Input: part model. Units: mm. Frame: model coordinates. Face numbers are marked on the shaded views. A direction names the side the tool comes from. Coordinates: 2 decimals unless noted, no trailing zeros. Loops run counter-clockwise (first coordinate to the right, second up) from the corner with the lowest first, then second, coordinate; pieces in that order, holes last. Notation, with made-up numbers: (81, 30.25) - (96, 30.25) arc R23 cw to (96, 51.25) - close; hole circle Ø10 at (11.5, 64). An arc over 180 degrees is marked (long way). Use a Markdown table: item, result. Add a question column.
1. Draft query along Y for the marked faces 4, 5, 6 and 7. Return one class per face: released by +Y, released by -Y, zero draft, split by the parting line, or undercut.
2. Contact query for flat-ended pins moving along their axis: P1, Ø2.5, axis at y = -2.5, z = -1, coming from the +X side; P2, Ø1.5, axis at y = -5.5, z = -2, coming from the -X side; P3, Ø16, axis at x = 11.5, y = -7.5, coming from the -Z side. Output: stop coordinate, or through.
3. Access query for the marked faces 1, 2 and 3. Directions: +Z, -Z, +X, -X, +Y, -Y. A direction counts if a zero-diameter tool reaches every point of the face in a straight line with its end or side. Return the directions, or none.
4. Section query A-A on z = -2.5. Return the cut outline in (x, y).
5. Section query B-B on x = -11.5. Return the cut outline in (y, z), then the cut area to 3 significant figures.
6. Ray query, L1, parallel to Y at x = 55.7, z = 1; L2, parallel to Z at x = -11.5, y = 7.5; L3, parallel to X at y = -3.5, z = -4.25. Return the intervals inside material, ascending. Write a range as [from, to].
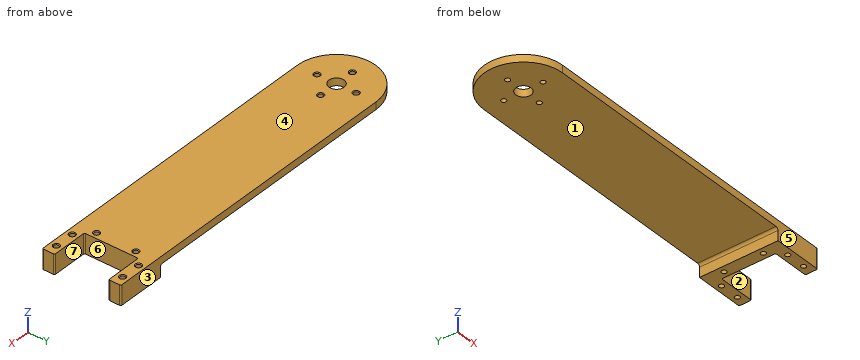
```python
from build123d import *

# Parameters (mm, degrees)
Y_KSEKLIK_EKSTR_ZYON1_DEPTH                    = 3
IZIM2_R                                        = 3.1
KES_EKSTR_ZYON1_DEPTH                          = 79.70196948
M2_D_Z_BA_L_MAKINE_VIDAS_IN_HAV_A1_D           = 2
M2_D_Z_BA_L_MAKINE_VIDAS_IN_HAV_A1_CSINK_D     = 2.6
M2_D_Z_BA_L_MAKINE_VIDAS_IN_HAV_A1_CSINK_ANGLE = 90
IZIM26_W                                       = 22.3
IZIM26_H                                       = 22
KES_EKSTR_ZYON4_DEPTH                          = 79.70196948
Y_KSEKLIK_EKSTR_ZYON3_DEPTH                    = 8
M2_D_Z_BA_L_MAKINE_VIDAS_IN_HAV_A2_D           = 2
M2_D_Z_BA_L_MAKINE_VIDAS_IN_HAV_A2_CSINK_D     = 2.6
M2_D_Z_BA_L_MAKINE_VIDAS_IN_HAV_A2_CSINK_ANGLE = 90
RADYUS1_R                                      = 1
IZIM38_W                                       = 7.3
IZIM38_H                                       = 32
KES_EKSTR_ZYON5_DEPTH                          = 80.050616696
RADYUS2_R                                      = 0.5


with BuildPart() as part:
    # Çizim1 → Yükseklik-Ekstrüzyon1 (new body)
    with BuildSketch(Plane.XY):
        with BuildLine():
            ThreePointArc((-61, 16), (-77, 0), (-61, -16))
            Line((-61, -16), (75, -16))
            Line((75, -16), (75, 16))
            Line((75, 16), (-61, 16))
        make_face()
    extrude(amount=Y_KSEKLIK_EKSTR_ZYON1_DEPTH)

    # Çizim2 → Kes-Ekstrüzyon1 (cut, through all)
    with BuildSketch(Plane.XY.offset(3)):
        with Locations((-61, 0)):
            Circle(IZIM2_R)
    extrude(amount=-KES_EKSTR_ZYON1_DEPTH, mode=Mode.SUBTRACT)

    # M2 Düz Başlı Makine Vidası İçin Havşa1 (through all)
    with Locations(Plane(origin=(-61, 8, 3), x_dir=(1, 0, 0), z_dir=(0, 0, 1))):
        with Locations((0, 0), (8, -8), (0, -16), (-8, -8)):
            CounterSinkHole(M2_D_Z_BA_L_MAKINE_VIDAS_IN_HAV_A1_D / 2, M2_D_Z_BA_L_MAKINE_VIDAS_IN_HAV_A1_CSINK_D / 2, counter_sink_angle=M2_D_Z_BA_L_MAKINE_VIDAS_IN_HAV_A1_CSINK_ANGLE)

    # Çizim26 → Kes-Ekstrüzyon4 (cut, through all)
    with BuildSketch(Plane.XY.offset(3)):
        with Locations((63.85, 0)):
            Rectangle(IZIM26_W, IZIM26_H)
    extrude(amount=-KES_EKSTR_ZYON4_DEPTH, mode=Mode.SUBTRACT)

    # Çizim33 → Yükseklik-Ekstrüzyon3 (add)
    with BuildSketch(Plane.XY.offset(3)):
        Polygon((75, 11), (75, 16), (47.7, 16), (47.7, -16), (75, -16), (75, -11), (52.7, -11), (52.7, 11), align=None)
    extrude(amount=-Y_KSEKLIK_EKSTR_ZYON3_DEPTH)

    # M2 Düz Başlı Makine Vidası İçin Havşa2 (through all)
    with Locations(Plane(origin=(71.7, 13.5, 3), x_dir=(1, 0, 0), z_dir=(0, 0, 1))):
        with Locations((0, 0), (-8, 0), (-16, 0), (-21.5, -5.5), (-21.5, -21.5), (-16, -27), (-8, -27), (0, -27)):
            CounterSinkHole(M2_D_Z_BA_L_MAKINE_VIDAS_IN_HAV_A2_D / 2, M2_D_Z_BA_L_MAKINE_VIDAS_IN_HAV_A2_CSINK_D / 2, counter_sink_angle=M2_D_Z_BA_L_MAKINE_VIDAS_IN_HAV_A2_CSINK_ANGLE)

    # Radyus1
    radyus1_edges = [part.edges().sort_by_distance(p)[0] for p in [
        (47.7, 0, 0),
    ]]
    fillet(radyus1_edges, radius=RADYUS1_R)

    # Çizim38 → Kes-Ekstrüzyon5 (cut, through all)
    with BuildSketch(Plane.XY.offset(3)):
        with Locations((71.35, 0)):
            Rectangle(IZIM38_W, IZIM38_H)
    extrude(amount=-KES_EKSTR_ZYON5_DEPTH, mode=Mode.SUBTRACT)

    # Radyus2
    radyus2_edges = [part.edges().sort_by_distance(p)[0] for p in [
        (67.7, -11, -1),
        (67.7, -16, -1),
        (67.7, 11, -1),
        (67.7, 16, -1),
        (52.7, -11, -1),
        (52.7, 11, -1),
    ]]
    fillet(radyus2_edges, radius=RADYUS2_R)


solid = part.part
```
Resolved:
| question | item | result |
|---|---|---|
| 1 | face 4 | zero draft |
| 1 | face 5 | released by -Y |
| 1 | face 6 | undercut |
| 1 | face 7 | undercut |
| 2 | P1 | x = 52.7 |
| 2 | P2 | x = 47.7 |
| 2 | P3 | z = 0 |
| 3 | face 1 | -Z, -X, +Y, -Y |
| 3 | face 2 | +Z, -Z, +X |
| 3 | face 3 | +Z, -Z, +X, -X, +Y |
| 4 | outline | (47.7, -16) - (67.2, -16) arc R0.5 ccw to (67.7, -15.5) - (67.7, -11.5) arc R0.5 ccw to (67.2, -11) - (53.2, -11) arc R0.5 cw to (52.7, -10.5) - (52.7, 10.5) arc R0.5 cw to (53.2, 11) - (67.2, 11) arc R0.5 ccw to (67.7, 11.5) - (67.7, 15.5) arc R0.5 ccw to (67.2, 16) - (47.7, 16) - close; hole circle Ø2 at (50.2, -8); hole circle Ø2 at (50.2, 8); hole circle Ø2 at (55.7, -13.5); hole circle Ø2 at (55.7, 13.5); hole circle Ø2 at (63.7, -13.5); hole circle Ø2 at (63.7, 13.5) |
| 5 | outline | (-16, 0) - (16, 0) - (16, 3) - (-16, 3) - close |
| 5 | area | 96.0 mm² |
| 6 | L1 | [-16, -14.5], [-12.5, -11], [11, 12.5], [14.5, 16] |
| 6 | L2 | [0, 3] |
| 6 | L3 | [47.7, 52.7] |
